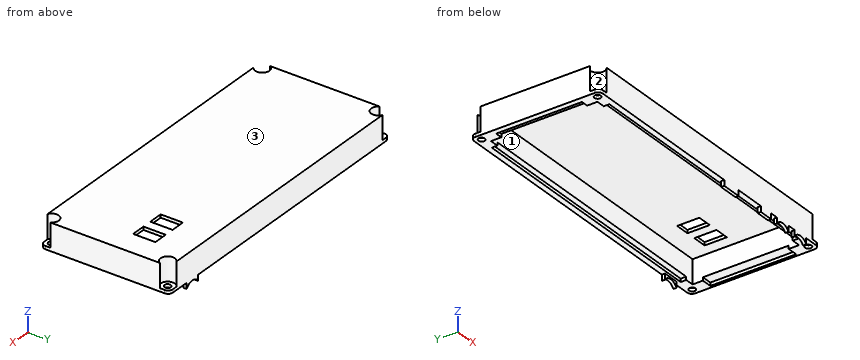
from build123d import *

# Parameters (mm, degrees)
BOX034_W          = 9
BOX034_H          = 2
BOX034_DEPTH      = 10
CYLINDER027_R     = 6
CYLINDER027_DEPTH = 10
BOX035_W          = 10
BOX035_H          = 2
BOX035_DEPTH      = 10
CYLINDER028_R     = 6
CYLINDER028_DEPTH = 10
BOX036_W          = 10
BOX036_H          = 2
BOX036_DEPTH      = 10
CYLINDER029_R     = 6
CYLINDER029_DEPTH = 10
BOX037_W          = 10
BOX037_H          = 2
BOX037_DEPTH      = 10
BOX033_W          = 12.5
BOX033_H          = 2
BOX033_DEPTH      = 10
BOX032_W          = 9
BOX032_H          = 14
BOX032_DEPTH      = 10
BOX031_W          = 9
BOX031_H          = 14
BOX031_DEPTH      = 10
CYLINDER023_R     = 4.5
CYLINDER023_DEPTH = 20
CYLINDER024_R     = 4.5
CYLINDER024_DEPTH = 20
CYLINDER025_R     = 4.5
CYLINDER025_DEPTH = 20
CYLINDER026_R     = 4.5
CYLINDER026_DEPTH = 20
CYLINDER020_R     = 2
CYLINDER020_DEPTH = 20
CYLINDER021_R     = 2
CYLINDER021_DEPTH = 20
CYLINDER022_R     = 2
CYLINDER022_DEPTH = 20
CYLINDER019_R     = 2
CYLINDER019_DEPTH = 20
BOX030_W          = 176
BOX030_H          = 67
BOX030_DEPTH      = 15
BOX029_W          = 165
BOX029_H          = 74
BOX029_DEPTH      = 2
BOX028_W          = 187
BOX028_H          = 54
BOX028_DEPTH      = 2
BOX027_W          = 192
BOX027_H          = 81
BOX027_DEPTH      = 17
FILLET001_R       = 3


with BuildPart() as cube018:
    # Box034 → Box034 (new body)
    with BuildSketch(Plane(origin=(139, 0, 17.5), x_dir=(1, 0, 0), z_dir=(0, 0, 1))):
        with Locations((4.5, 1)):
            Rectangle(BOX034_W, BOX034_H)
    extrude(amount=BOX034_DEPTH)


with BuildPart() as cylinder027:
    # Cylinder027 → Cylinder027 (new body)
    with BuildSketch(Plane(origin=(158, -4, 13), x_dir=(1, 0, 0), z_dir=(0, 1, 0))):
        Circle(CYLINDER027_R)
    extrude(amount=CYLINDER027_DEPTH)


with BuildPart() as cut010:
    # Box035 → Box035 (new body)
    with BuildSketch(Plane(origin=(153, 0, 14.5), x_dir=(1, 0, 0), z_dir=(0, 0, 1))):
        with Locations((5, 1)):
            Rectangle(BOX035_W, BOX035_H)
    extrude(amount=BOX035_DEPTH)

    # Cut010: cut Cylinder027
    add(cylinder027.part, mode=Mode.SUBTRACT)


with BuildPart() as cut010_1:
    # Cut010 placement: moved
    add(cut010.part.moved(Location((0, 0, 1))))


with BuildPart() as cylinder028:
    # Cylinder028 → Cylinder028 (new body)
    with BuildSketch(Plane(origin=(158, -4, 13), x_dir=(1, 0, 0), z_dir=(0, 1, 0))):
        Circle(CYLINDER028_R)
    extrude(amount=CYLINDER028_DEPTH)


with BuildPart() as cut011:
    # Box036 → Box036 (new body)
    with BuildSketch(Plane(origin=(153, 0, 14.5), x_dir=(1, 0, 0), z_dir=(0, 0, 1))):
        with Locations((5, 1)):
            Rectangle(BOX036_W, BOX036_H)
    extrude(amount=BOX036_DEPTH)

    # Cut011: cut Cylinder028
    add(cylinder028.part, mode=Mode.SUBTRACT)


with BuildPart() as cut011_1:
    # Cut011 placement: moved
    add(cut011.part.moved(Location((12, 79, 1))))


with BuildPart() as cylinder029:
    # Cylinder029 → Cylinder029 (new body)
    with BuildSketch(Plane(origin=(158, -4, 13), x_dir=(1, 0, 0), z_dir=(0, 1, 0))):
        Circle(CYLINDER029_R)
    extrude(amount=CYLINDER029_DEPTH)


with BuildPart() as cut012:
    # Box037 → Box037 (new body)
    with BuildSketch(Plane(origin=(153, 0, 14.5), x_dir=(1, 0, 0), z_dir=(0, 0, 1))):
        with Locations((5, 1)):
            Rectangle(BOX037_W, BOX037_H)
    extrude(amount=BOX037_DEPTH)

    # Cut012: cut Cylinder029
    add(cylinder029.part, mode=Mode.SUBTRACT)


with BuildPart() as cut012_1:
    # Cut012 placement: moved
    add(cut012.part.moved(Location((15.5, 0, 1))))


with BuildPart() as coverholes:
    # Box033 → Box033 (new body)
    with BuildSketch(Plane(origin=(107, 0, 17.5), x_dir=(1, 0, 0), z_dir=(0, 0, 1))):
        with Locations((6.25, 1)):
            Rectangle(BOX033_W, BOX033_H)
    extrude(amount=BOX033_DEPTH)

    # Compound002: union Cube018, Cut010, Cut011, Cut012
    add(cube018.part)
    add(cut010_1.part)
    add(cut011_1.part)
    add(cut012_1.part)


with BuildPart() as switch_placement_hole001:
    # Box032 → Box032 (new body)
    with BuildSketch(Plane(origin=(150.5, 47, 31), x_dir=(1, 0, 0), z_dir=(0, 0, 1))):
        with Locations((4.5, 7)):
            Rectangle(BOX032_W, BOX032_H)
    extrude(amount=BOX032_DEPTH)


with BuildPart() as compound001:
    # Box031 → Box031 (new body)
    with BuildSketch(Plane(origin=(165.5, 47, 31), x_dir=(1, 0, 0), z_dir=(0, 0, 1))):
        with Locations((4.5, 7)):
            Rectangle(BOX031_W, BOX031_H)
    extrude(amount=BOX031_DEPTH)

    # Compound001: union Switch Placement Hole001
    add(switch_placement_hole001.part)


with BuildPart() as cylinder023:
    # Cylinder023 → Cylinder023 (new body)
    with BuildSketch(Plane(origin=(2, 77, 0), x_dir=(1, 0, 0), z_dir=(0, 0, 1))):
        Circle(CYLINDER023_R)
    extrude(amount=CYLINDER023_DEPTH)


with BuildPart() as cylinder024:
    # Cylinder024 → Cylinder024 (new body)
    with BuildSketch(Plane(origin=(186, 77, 0), x_dir=(1, 0, 0), z_dir=(0, 0, 1))):
        Circle(CYLINDER024_R)
    extrude(amount=CYLINDER024_DEPTH)


with BuildPart() as cylinder025:
    # Cylinder025 → Cylinder025 (new body)
    with BuildSketch(Plane(origin=(186, 4, 0), x_dir=(1, 0, 0), z_dir=(0, 0, 1))):
        Circle(CYLINDER025_R)
    extrude(amount=CYLINDER025_DEPTH)


with BuildPart() as fusion015:
    # Cylinder026 → Cylinder026 (new body)
    with BuildSketch(Plane(origin=(2, 4, 0), x_dir=(1, 0, 0), z_dir=(0, 0, 1))):
        Circle(CYLINDER026_R)
    extrude(amount=CYLINDER026_DEPTH)

    # Fusion015: union Cylinder023, Cylinder024, Cylinder025
    add(cylinder023.part)
    add(cylinder024.part)
    add(cylinder025.part)


with BuildPart() as fusion015_1:
    # Fusion015 placement: moved
    add(fusion015.part.moved(Location((0, 0, 23))))


with BuildPart() as cylinder020:
    # Cylinder020 → Cylinder020 (new body)
    with BuildSketch(Plane(origin=(2, 77, 0), x_dir=(1, 0, 0), z_dir=(0, 0, 1))):
        Circle(CYLINDER020_R)
    extrude(amount=CYLINDER020_DEPTH)


with BuildPart() as cylinder021:
    # Cylinder021 → Cylinder021 (new body)
    with BuildSketch(Plane(origin=(186, 77, 0), x_dir=(1, 0, 0), z_dir=(0, 0, 1))):
        Circle(CYLINDER021_R)
    extrude(amount=CYLINDER021_DEPTH)


with BuildPart() as cylinder022:
    # Cylinder022 → Cylinder022 (new body)
    with BuildSketch(Plane(origin=(186, 4, 0), x_dir=(1, 0, 0), z_dir=(0, 0, 1))):
        Circle(CYLINDER022_R)
    extrude(amount=CYLINDER022_DEPTH)


with BuildPart() as fusion014:
    # Cylinder019 → Cylinder019 (new body)
    with BuildSketch(Plane(origin=(2, 4, 0), x_dir=(1, 0, 0), z_dir=(0, 0, 1))):
        Circle(CYLINDER019_R)
    extrude(amount=CYLINDER019_DEPTH)

    # Fusion014: union Cylinder020, Cylinder021, Cylinder022
    add(cylinder020.part)
    add(cylinder021.part)
    add(cylinder022.part)


with BuildPart() as fusion014_1:
    # Fusion014 placement: moved
    add(fusion014.part.moved(Location((0, 0, 18))))


with BuildPart() as cube016:
    # Box030 → Box030 (new body)
    with BuildSketch(Plane(origin=(6, 7, 21), x_dir=(1, 0, 0), z_dir=(0, 0, 1))):
        with Locations((88, 33.5)):
            Rectangle(BOX030_W, BOX030_H)
    extrude(amount=BOX030_DEPTH)


with BuildPart() as cube015:
    # Box029 → Box029 (new body)
    with BuildSketch(Plane(origin=(11.5, 3.5, 21), x_dir=(1, 0, 0), z_dir=(0, 0, 1))):
        with Locations((82.5, 37)):
            Rectangle(BOX029_W, BOX029_H)
    extrude(amount=BOX029_DEPTH)


with BuildPart() as obj1:
    # Box028 → Box028 (new body)
    with BuildSketch(Plane(origin=(1.5, 13.5, 21), x_dir=(1, 0, 0), z_dir=(0, 0, 1))):
        with Locations((93.5, 27)):
            Rectangle(BOX028_W, BOX028_H)
    extrude(amount=BOX028_DEPTH)

    # Fusion013: union Cube015
    add(cube015.part)


with BuildPart() as cover:
    # Box027 → Box027 (new body)
    with BuildSketch(Plane(origin=(-2, 0, 21), x_dir=(1, 0, 0), z_dir=(0, 0, 1))):
        with Locations((96, 40.5)):
            Rectangle(BOX027_W, BOX027_H)
    extrude(amount=BOX027_DEPTH)

    # Fillet001
    fillet001_edges = [cover.edges().sort_by_distance(p)[0] for p in [
        (-2, 0, 29.5),
        (-2, 81, 29.5),
        (190, 0, 29.5),
        (190, 81, 29.5),
    ]]
    fillet(fillet001_edges, radius=FILLET001_R)

    # Cut005: cut obj1
    add(obj1.part, mode=Mode.SUBTRACT)

    # Cut006: cut Cube016
    add(cube016.part, mode=Mode.SUBTRACT)

    # Cut007: cut Fusion014
    add(fusion014_1.part, mode=Mode.SUBTRACT)

    # Cut008: cut Fusion015
    add(fusion015_1.part, mode=Mode.SUBTRACT)

    # Cut009: cut Compound001
    add(compound001.part, mode=Mode.SUBTRACT)

    # Fusion016: union CoverHoles
    add(coverholes.part)


solid = cover.part
For this review, take the finished solid that the model builds, in its own axes (mm). Face numbers are marked on the shaded views. A direction names the side the tool comes from. Round coordinates to 2 decimals unless told otherwise and drop trailing zeros. Loops run counter-clockwise (first coordinate to the right, second up) from the corner with the lowest first, then second, coordinate; pieces in that order, holes last. Notation, with made-up numbers: (43.5, 65.5) - (65.5, 65.5) arc R7 ccw to (65.5, 69.5) - close; hole circle Ø2 at (52.25, 54.25). An arc over 180 degrees is marked (long way). Put each result on its own line as item: value. Start each with the question number.
1. Consider section C-C on x = 128. State the section outline as (y, z) points.
2. Consider section D-D on z = 28.75. State the section outline as (x, y) points.
3. For the marked faces 1, 2 and 3, list the 3-axis set-ups (+Z, -Z, +X, -X, +Y, -Y) from which the entire face can be reached by the end or side of a thin tool; tool diameter is ignored.
4. For probe 1 along X at (y, z) = (77, 22); probe 2 along Y at (x, z) = (186, 21.5); probe 3 along X at (y, z) = (27.5, 23.25), list the stretches that pass through material, from the lowest coordinate up. Write a range as [from, to].
5. Insertion check: P1, Ø8, axis at x = 136, y = 59.5, coming from the -Z side; P2, Ø2, axis at y = 79.5, z = 19.5, coming from the -X side; P3, Ø1, axis at y = 1, z = 19, coming from the +X side; P4, Ø2.5, axis at x = 2, y = 77, coming from the -Z side. Each pin has a flat end and moves straight along its axis. Give the tip position at first contact, or say it passes through.
6. Consider section B-B on y = 51.5. State the section outline as (x, z) points.
7. Consider section A-A on y = 10.5. State the section outline as (x, z) points, plus the area to 3 significant figures.
Result sheet:
1. outline: (0, 21) - (3.5, 21) - (3.5, 23) - (7, 23) - (7, 36) - (74, 36) - (74, 23) - (77.5, 23) - (77.5, 21) - (81, 21) - (81, 38) - (0, 38) - close
2. outline: (-2, 6.06) arc R4.5 cw (long way) to (4.06, 0) - (183.94, 0) arc R4.5 cw (long way) to (190, 6.06) - (190, 74.94) arc R4.5 cw (long way) to (183.94, 81) - (4.06, 81) arc R4.5 cw (long way) to (-2, 74.94) - close; hole (6, 7) - (182, 7) - (182, 74) - (6, 74) - close
3. face 1: -Z
3. face 2: +Z
3. face 3: +Z, +X, -X, +Y, -Y
4. probe 1: [-2, 0], [4, 11.5], [176.5, 184], [188, 190]
4. probe 2: [0, 2], [6, 13.5], [67.5, 75], [79, 81]
4. probe 3: [-2, 6], [182, 190]
5. P1: z = 36
5. P2: x = 165
5. P3: x = 178.5
5. P4: through
6. outline: (-2, 21) - (1.5, 21) - (1.5, 23) - (6, 23) - (6, 36) - (150.5, 36) - (150.5, 38) - (-2, 38) - close; (159.5, 36) - (165.5, 36) - (165.5, 38) - (159.5, 38) - close; (174.5, 36) - (182, 36) - (182, 23) - (188.5, 23) - (188.5, 21) - (190, 21) - (190, 38) - (174.5, 38) - close
7. outline: (-2, 21) - (6, 21) - (6, 36) - (182, 36) - (182, 21) - (190, 21) - (190, 38) - (-2, 38) - close
7. area: 624 mm^2
